Source: three-view drawing plus pictorial views. Frame: mm from the lowest corner of the part. A direction names the side the tool comes from. Give positions to 0.01 mm unless a question says otherwise; leave off trailing zeros. Write each loop counter-clockwise with the first axis right and the second up, starting at its lowest first coordinate (ties: lowest second). Pieces come first, ordered by that corner, then holes.
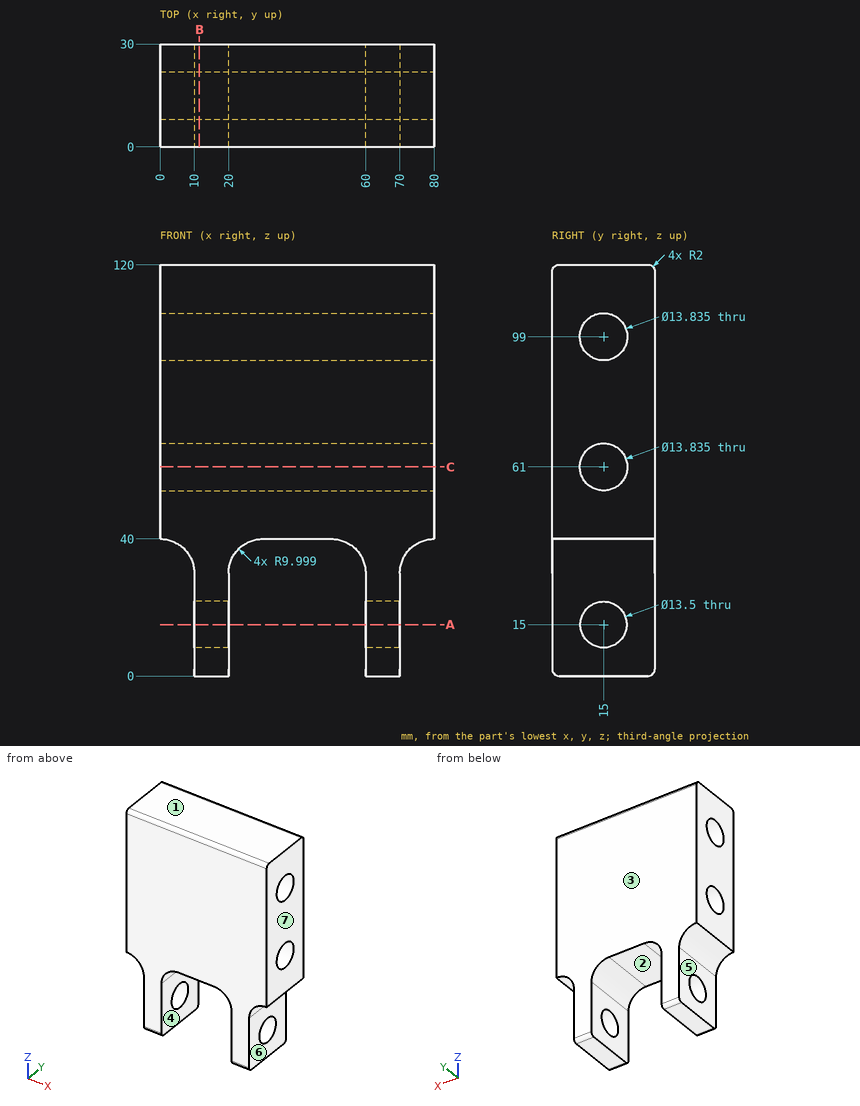
Q1. Pull-direction query (Z, two-part tool) for the marked faces 1, 2 and 3; classes: released by +Z, released by -Z, zero draft, split by the parting line, or undercut.
Filled sheet:
face 1: released by +Z
face 2: released by -Z
face 3: zero draft
Q2. Section B-B on x = 11.5. Count the separate pieces of the cut face and the enclosed holes in it, plus the area to 3 significant figures.
Filled sheet:
separate pieces: 1
enclosed holes: 3
area: 3,150 mm2
Q3. Section A-A on z = 15. Output: boundary loops of the cut face in (x, y).
Filled sheet:
outline: (10, 0) - (20, 0) - (20, 8.25) - (10, 8.25) - close; (10, 21.75) - (20, 21.75) - (20, 30) - (10, 30) - close; (60, 0) - (70, 0) - (70, 8.25) - (60, 8.25) - close; (60, 21.75) - (70, 21.75) - (70, 30) - (60, 30) - close
Q4. Ray query, line 1 along Z through (x, y) = (67.5, 15); line 2 along Y through (x, z) = (17.75, 15); line 3 along Z through (x, y) = (57.5, 15) (1 decimal). Return the intervals inside material, ascending.
Filled sheet:
line 1: z = 0 to 8.25, 21.75 to 54.08, 67.92 to 92.08, 105.92 to 120
line 2: y = 0 to 8.25, 21.75 to 30
line 3: z = 36.6 to 54.1, 67.9 to 92.1, 105.9 to 120
Q5. Access query for the marked faces 4, 5, 6 and 7. Directions: +Z, -Z, +X, -X, +Y, -Y. A direction counts if a zero-diameter tool reaches every point of the face in a straight line with its end or side. Return the directions, or none.
Filled sheet:
face 4: -Z, +Y, -Y
face 5: -Z, -X, +Y, -Y
face 6: -Z, +X, +Y, -Y
face 7: +Z, -Z, +X, +Y, -Y
Q6. Section C-C on z = 61. Output: boundary loops of the cut face in (x, y).
Filled sheet:
outline: (0, 0) - (80, 0) - (80, 8.08) - (0, 8.08) - close; (0, 21.92) - (80, 21.92) - (80, 30) - (0, 30) - close
Q7. Pin query (flat end, axial travel): P1, Ø11, axis at y = 15, z = 15, coming from the -X side; P2, Ø8, axis at x = 16.5, z = 24, coming from the -Y side; P3, Ø8, axis at x = 28, y = 14.5, coming from the -Z side; P4, Ø16, axis at x = 45, y = 9.5, coming from the -Z side. Return the tip coordinate at first contact, or that it passes through.
Filled sheet:
P1: passes through
P2: stops at y = 0
P3: stops at z = 38
P4: stops at z = 39.54
